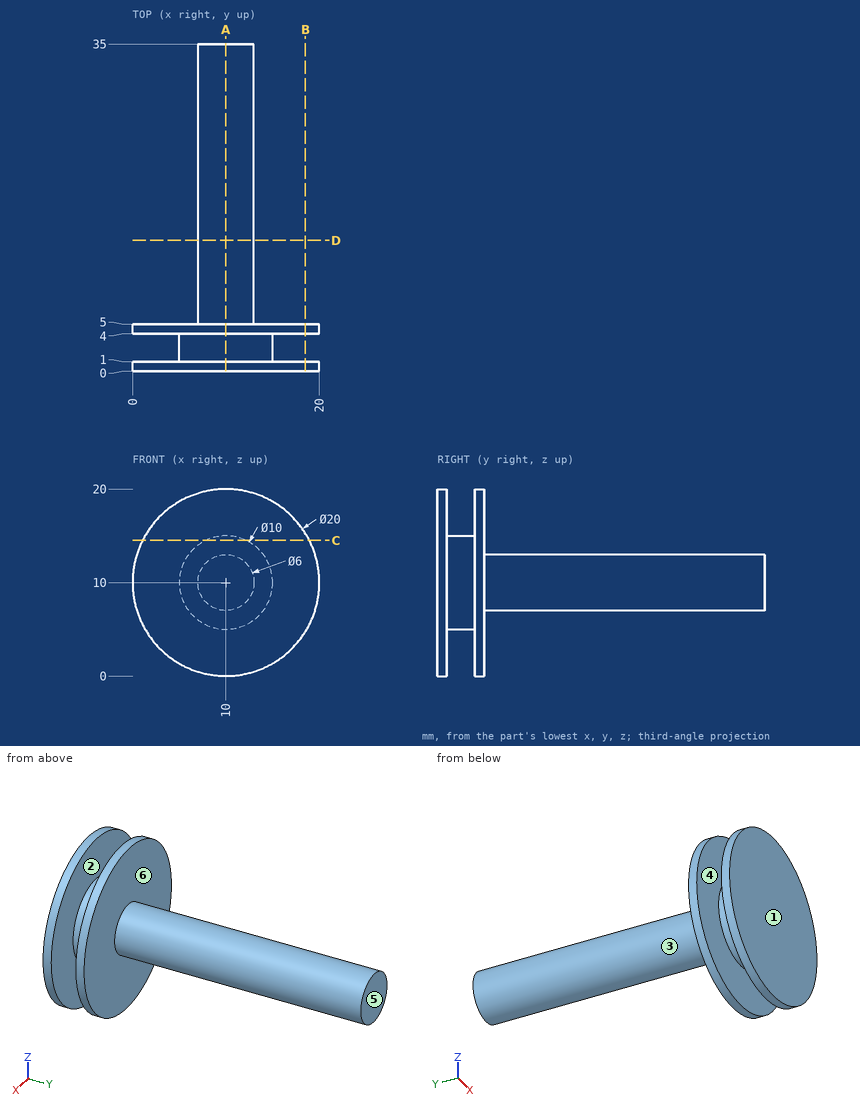
Input: dimensioned drawing with shaded views. Units: mm. Origin: part minimum x, y, z. A direction names the side the tool comes from. Round coordinates to 2 decimals unless told otherwise and drop trailing zeros. Loops run counter-clockwise (first coordinate to the right, second up) from the corner with the lowest first, then second, coordinate; pieces in that order, holes last. Notation, with made-up numbers: (72, 60) -> (129, 60) arc R20 ccw to (129, 66) -> close; hole circle Ø10 at (83.25, 59.5). An arc over 180 degrees is marked (long way). Answer as a JSON object with one key per item and string values. Group by question number.
Q1. Ray query, line 1 (Y direction, x = 2, z = 13.25); line 2 (Z direction, x = 10, y = 29); line 3 (X direction, y = 31, z = 8). Return the intervals inside material, ascending. Write a range as from..to.
Q2. Section query D-D (y = 14). Output: boundary loops of the cut face in (x, z).
Q3. Access query for the marked faces 4, 5 and 6. Directions: +Z, -Z, +X, -X, +Y, -Y. A direction counts if a zero-diameter tool reaches every point of the face in a straight line with its end or side. Return the directions, or none.
Q4. Section query B-B (x = 18.5). Output: boundary loops of the cut face in (y, z), plus the area to 3 significant figures.
Q5. Section query C-C (z = 14.5). Output: boundary loops of the cut face in (x, y), plus the area to 3 significant figures.
Q6. Mould query, pull axis Y, two halves, no side actions, for the marked faces 1, 2 and 3. Classes: pulls with the +Y half, pulls with the -Y half, needs draft (parallel to the pull), parting line crosses it, or undercut.
Q7. Section query A-A (x = 10). Output: boundary loops of the cut face in (y, z).
Q8. Contact query for flat-ended pins moving along their axis: P1, Ø4, axis at x = 11.5, y = 31, coming from the -Z side; P2, Ø3, axis at y = 27.5, z = 13, coming from the -X side; P3, Ø1, axis at y = 4, z = 4, coming from the -X side. Output: stop coordinate, or through.
Completed:
{
 "1": {"line 1": "0..1, 4..5", "line 2": "7..13", "line 3": "7.76..12.24"},
 "2": {"outline": "circle Ø6 at (10, 10)"},
 "3": {"face 4": "none", "face 5": "+Z, -Z, +X, -X, +Y", "face 6": "+Y"},
 "4": {"outline": "(0, 4.73) -> (1, 4.73) -> (1, 15.27) -> (0, 15.27) -> close; (4, 4.73) -> (5, 4.73) -> (5, 15.27) -> (4, 15.27) -> close", "area": "21.1 mm²"},
 "5": {"outline": "(1.07, 0) -> (18.93, 0) -> (18.93, 1) -> (12.18, 1) -> (12.18, 4) -> (18.93, 4) -> (18.93, 5) -> (1.07, 5) -> (1.07, 4) -> (7.82, 4) -> (7.82, 1) -> (1.07, 1) -> close", "area": "48.8 mm²"},
 "6": {"face 1": "pulls with the -Y half", "face 2": "undercut", "face 3": "needs draft"},
 "7": {"outline": "(0, 0) -> (1, 0) -> (1, 5) -> (4, 5) -> (4, 0) -> (5, 0) -> (5, 7) -> (35, 7) -> (35, 13) -> (5, 13) -> (5, 20) -> (4, 20) -> (4, 15) -> (1, 15) -> (1, 20) -> (0, 20) -> close"},
 "8": {"P1": "z = 7", "P2": "x = 7.4", "P3": "x = 1.65"}
}
